Read the model definition and answer for the solid it produces. Units are mm, in the model's axes. A direction names the side the tool comes from. Give positions to 0.01 mm unless a question says otherwise; leave off trailing zeros. Write each loop counter-clockwise with the first axis right and the second up, starting at its lowest first coordinate (ties: lowest second). Pieces come first, ordered by that corner, then holes. Notation, with made-up numbers: (43.5, -16) -> (50.5, -16) arc R26 ccw to (50.5, 16) -> close; hole circle Ø6 at (-14, -34.75). An arc over 180 degrees is marked (long way). Use a Markdown table: item, result.
from build123d import *

# Parameters (mm, degrees)
F0_W      = 838.2
F0_H      = 762
F1_DEPTH  = 1676.4
F2_W      = 838.2
F2_H      = 533.4
F2_W_2    = 38.1
F2_H_2    = 203.2
F3_DEPTH  = 50.8
F4_R      = 12.7
F5_DEPTH  = 50.8
F6_R      = 12.69999
F7_W      = 40.6822860241
F7_H      = 212.2554779053
F8_DEPTH  = 38.1
F9_SIZE   = 5.08
F10_W     = 38.9135181904
F10_H     = 413.8980805874
F11_DEPTH = 38.1
F12_SIZE  = 5.08


# Not quite as in the source:
# - a fillet or chamfer is up to 0.001 mm smaller than in the source, because OpenCascade refuses the exact size


with BuildPart() as f1:
    # F0 (on Top) → F1 (new body)
    with BuildSketch(Plane.XY):
        Rectangle(F0_W, F0_H)
    extrude(amount=F1_DEPTH)

    # F2 (on face) → F3 (join)
    with BuildSketch(Plane.XZ.offset(381)):
        with Locations((0, 1409.7)):
            Rectangle(F2_W, F2_H)
        with Locations((-346.277383852, 1415.0833574295)):
            Rectangle(F2_W_2, F2_H_2, mode=Mode.SUBTRACT)
        with Locations((-346.277383852, 1415.0833574295)):
            Rectangle(F2_W_2, F2_H_2)
    extrude(amount=F3_DEPTH)

    # F4
    f4_edges = [f1.edges().sort_by_distance(p)[0] for p in [
        (0, -431.8, 1676.4),
        (-419.1, -431.8, 1409.7),
        (0, -431.8, 1143),
        (419.1, -431.8, 1409.7),
    ]]
    fillet(f4_edges, radius=F4_R)

    # F5 (add): a face of the model
    f5_faces = [f1.faces().sort_by_distance(p)[0] for p in [
        (0, -381, 571.5),
    ]]
    extrude(f5_faces, amount=F5_DEPTH)

    # F6 (radius 12.7 in the source; OpenCascade refuses exactly that, so slightly less here)
    f6_edges = [f1.edges().sort_by_distance(p)[0] for p in [
        (0, -431.8, 0),
        (419.1, -431.8, 571.5),
        (0, -431.8, 1143),
        (-419.1, -431.8, 571.5),
    ]]
    fillet(f6_edges, radius=F6_R)

    # F7 (on face) → F8 (join)
    with BuildSketch(Plane.XZ.offset(431.8)):
        with Locations((-345.143482089, 1418.1935787201)):
            Rectangle(F7_W, F7_H)
    extrude(amount=F8_DEPTH)

    # F9
    f9_edges = [f1.edges().sort_by_distance(p)[0] for p in [
        (-345.143482, -469.9, 1524.321318),
        (-365.484625, -469.9, 1418.193579),
        (-345.143482, -469.9, 1312.06584),
        (-324.802339, -469.9, 1418.193579),
    ]]
    chamfer(f9_edges, length=F9_SIZE)

    # F10 (on face) → F11 (join)
    with BuildSketch(Plane.XZ.offset(431.8)):
        with Locations((-346.0278660059, 616.92930758)):
            Rectangle(F10_W, F10_H)
    extrude(amount=F11_DEPTH)

    # F12
    f12_edges = [f1.edges().sort_by_distance(p)[0] for p in [
        (-346.027866, -469.9, 823.878348),
        (-365.484625, -469.9, 616.929308),
        (-346.027866, -469.9, 409.980267),
        (-326.571107, -469.9, 616.929308),
    ]]
    chamfer(f12_edges, length=F12_SIZE)


solid = f1.part
Item 1: A cutting plane is placed at D-D (z = 266.5). Give the vertices of the cut face in (x, y).
Return value:
| item | result |
|---|---|
| outline | (-419.1, -419.1) arc R12.7 ccw to (-406.4, -431.8) -> (406.4, -431.8) arc R12.7 ccw to (419.1, -419.1) -> (419.1, 381) -> (-419.1, 381) -> close |
Item 2: A straight line is drawn through the part: line 1 along Y through (x, z) = (-184, 1167.5). Find the intervals that lie inside material, in ascending order. Write a range as [from, to].
Return value:
| item | result |
|---|---|
| line 1 | [-431.8, 381] |
Item 3: A cutting plane is placed at A-A (x = 2.5). Give the vertices of the cut face in (y, z), then the cut area to 3 significant figures.
Return value:
| item | result |
|---|---|
| outline | (-431.8, 12.7) arc R12.7 ccw to (-419.1, 0) -> (381, 0) -> (381, 1676.4) -> (-419.1, 1676.4) arc R12.7 ccw to (-431.8, 1663.7) -> (-431.8, 1155.7) arc R12.7 ccw to (-419.1, 1143) arc R12.7 ccw to (-431.8, 1130.3) -> close |
| area | 1,360,000 mm^2 |
Item 4: Each of these flat-tipped pins is pushed along its axis until it touches: P1, Ø16.5, axis at x = -336.5, y = -452, coming from the +Z side; P2, Ø16.5, axis at y = -456, z = 618.5, coming from the -X side; P3, Ø16.5, axis at x = -352.5, y = -441.5, coming from the -Z side. Where does it stop, or does it pass through?
Return value:
| item | result |
|---|---|
| P1 | z = 1524.32 |
| P2 | x = -365.48 |
| P3 | z = 409.98 |
Item 5: A cutting plane is placed at B-B (z = 1377). Give the vertices of the cut face in (x, y), then the cut area to 3 significant figures.
Return value:
| item | result |
|---|---|
| outline | (-419.1, -419.1) arc R12.7 ccw to (-406.4, -431.8) -> (-365.48, -431.8) -> (-365.48, -464.82) -> (-360.4, -469.9) -> (-329.88, -469.9) -> (-324.8, -464.82) -> (-324.8, -431.8) -> (406.4, -431.8) arc R12.7 ccw to (419.1, -419.1) -> (419.1, 381) -> (-419.1, 381) -> close |
| area | 683,000 mm^2 |
Item 6: A tool of negligible diameter and unlimited length cuts with its end or side. For faces 4 (the face through (-324.802, -448, 1417)), 5 (the face through (-346, -448, 823.878)), 6 (the face through (-365.485, -448, 614)), 7 (the face through (-345, -448, 1524.321)), 8 (the face through (-346, -448, 409.98)), from which of +Z, -Z, +X, -X, +Y, -Y can it reach the whole face along a straight path? Write none if from no direction.
Return value:
| item | result |
|---|---|
| face 4 | +Z, -Z, +X, -Y |
| face 5 | +X, -X, -Y |
| face 6 | +Z, -Z, -X, -Y |
| face 7 | +Z, +X, -X, -Y |
| face 8 | -Z, +X, -X, -Y |
Item 7: A cutting plane is placed at C-C (z = 768). Give the vertices of the cut face in (x, y), then the cut area to 3 significant figures.
Return value:
| item | result |
|---|---|
| outline | (-419.1, -419.1) arc R12.7 ccw to (-406.4, -431.8) -> (-365.48, -431.8) -> (-365.48, -464.82) -> (-360.4, -469.9) -> (-331.65, -469.9) -> (-326.57, -464.82) -> (-326.57, -431.8) -> (406.4, -431.8) arc R12.7 ccw to (419.1, -419.1) -> (419.1, 381) -> (-419.1, 381) -> close |
| area | 683,000 mm^2 |
Item 8: For a pull along Z with two mould halves and no side action, classify faces 1 (the face through (419.1, -13, 826)), 2 (the face through (-345, -448, 1312.066)), 3 (the face through (-6, -13, 1676.4)) as +Z half, -Z half, draft (parallel to the pull), parting line (faces both ways), or undercut.
Return value:
| item | result |
|---|---|
| face 1 | draft |
| face 2 | undercut |
| face 3 | +Z half |
